Geometry: final body of the model. Coordinates: model frame, mm. Face numbers are marked on the shaded views. Give positions to 0.01 mm unless a question says otherwise; leave off trailing zeros. Loops run counter-clockwise (first coordinate to the right, second up) from the corner with the lowest first, then second, coordinate; pieces in that order, holes last. Notation, with made-up numbers: M 87,51 L 140,51 A10 ccw 140,57 Z; hole C 62,42 d5. An arc over 180 degrees is marked long. Put each result on its own line as item: value.
```python
from build123d import *

# Parameters (mm, degrees)
F1_DEPTH = 5


with BuildPart() as f1:
    # F0 (on Top) → F1 (new body)
    with BuildSketch(Plane.XY):
        with BuildLine():
            Line((21.70305, 29.797339), (-28.29695, 29.797339))
            Line((-28.29695, 29.797339), (-28.29695, 8.297339))
            ThreePointArc((-28.29695, 8.297339), (-27.85761, 7.236679), (-26.79695, 6.797339))
            Line((-26.79695, 6.797339), (-26.079591, 6.797339))
            ThreePointArc((-26.079591, 6.797339), (-25.439988, 6.940538), (-24.922507, 7.342794))
            ThreePointArc((-24.922507, 7.342794), (-17.83695, 4.797339), (-24.922507, 2.251885))
            ThreePointArc((-24.922507, 2.251885), (-25.439988, 2.65414), (-26.079591, 2.797339))
            Line((-26.079591, 2.797339), (-26.79695, 2.797339))
            ThreePointArc((-26.79695, 2.797339), (-27.85761, 2.358), (-28.29695, 1.297339))
            Line((-28.29695, 1.297339), (-28.29695, -20.202661))
            Line((-28.29695, -20.202661), (21.70305, -20.202661))
            Line((21.70305, -20.202661), (21.70305, 1.297339))
            ThreePointArc((21.70305, 1.297339), (22.14239, 2.358), (23.20305, 2.797339))
            Line((23.20305, 2.797339), (23.920409, 2.797339))
            ThreePointArc((23.920409, 2.797339), (24.560012, 2.65414), (25.077493, 2.251885))
            ThreePointArc((25.077493, 2.251885), (29.515413, 1.032885), (32.16305, 4.797339))
            ThreePointArc((32.16305, 4.797339), (29.515413, 8.561793), (25.077493, 7.342794))
            ThreePointArc((25.077493, 7.342794), (24.560012, 6.940538), (23.920409, 6.797339))
            Line((23.920409, 6.797339), (23.20305, 6.797339))
            ThreePointArc((23.20305, 6.797339), (22.14239, 7.236679), (21.70305, 8.297339))
            Line((21.70305, 8.297339), (21.70305, 29.797339))
        make_face()
    extrude(amount=F1_DEPTH)


solid = f1.part
```
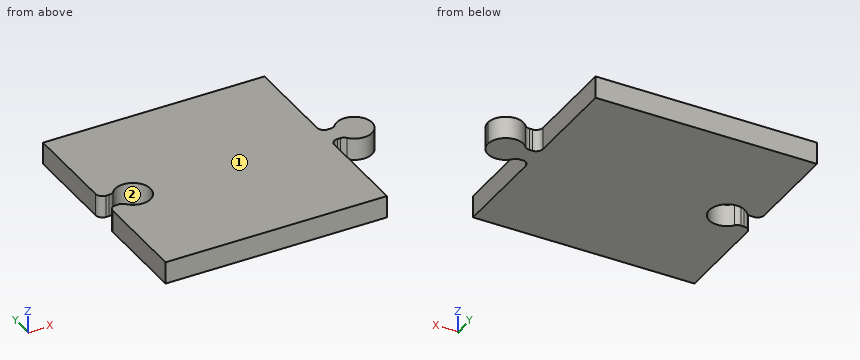
Item 1: Pin query (flat end, axial travel): pin 1 Ø1.5 at (y, z) = (22.5, 2) entering from +X; pin 2 Ø5 at (x, y) = (-21.84, 4.8) entering from -Z. Return the tip coordinate at first contact, or that it passes through.
Output values:
pin 1: x = 21.7
pin 2: through
Item 2: Section B-B on x = -18.5. Output: boundary loops of the cut face in (y, z), then the cut area to 3 significant figures.
Output values:
outline: M -20.2,0 L 2.59,0 L 2.59,5 L -20.2,5 Z; M 7,0 L 29.8,0 L 29.8,5 L 7,5 Z
area: 228 mm²
Item 3: Section A-A on z = 4.2. Output: boundary loops of the cut face in (x, y), then the cut area to 3 significant figures.
Output values:
outline: M -28.3,-20.2 L 21.7,-20.2 L 21.7,1.3 A1.5 cw 23.2,2.8 L 23.92,2.8 A1.5 cw 25.08,2.25 A4 ccw long 25.08,7.34 A1.5 cw 23.92,6.8 L 23.2,6.8 A1.5 cw 21.7,8.3 L 21.7,29.8 L -28.3,29.8 L -28.3,8.3 A1.5 ccw -26.8,6.8 L -26.08,6.8 A1.5 ccw -24.92,7.34 A4 cw long -24.92,2.25 A1.5 ccw -26.08,2.8 L -26.8,2.8 A1.5 ccw -28.3,1.3 Z
area: 2,500 mm²
Item 4: Mould query, pull axis X, two halves, no side actions, for the marked faces 1 and 2. Classes: pulls with the +X half, pulls with the -X half, needs draft (parallel to the pull), parting line crosses it, or undercut.
Output values:
face 1: needs draft
face 2: undercut
Item 5: Line query: probe 1 along X at (y, z) = (9, 1.5); probe 2 along Y at (x, z) = (28.5, 2.25); probe 3 along Y at (x, z) = (25.5, 3.9). Output: solid intervals per line, ascending. Write a range as [from, to].
Output values:
probe 1: [-28.3, 21.7]
probe 2: [0.81, 8.78]
probe 3: [1.81, 7.78]
Item 6: Section C-C on y = 20. Output: boundary loops of the cut face in (x, z).
Output values:
outline: M -28.3,0 L 21.7,0 L 21.7,5 L -28.3,5 Z
